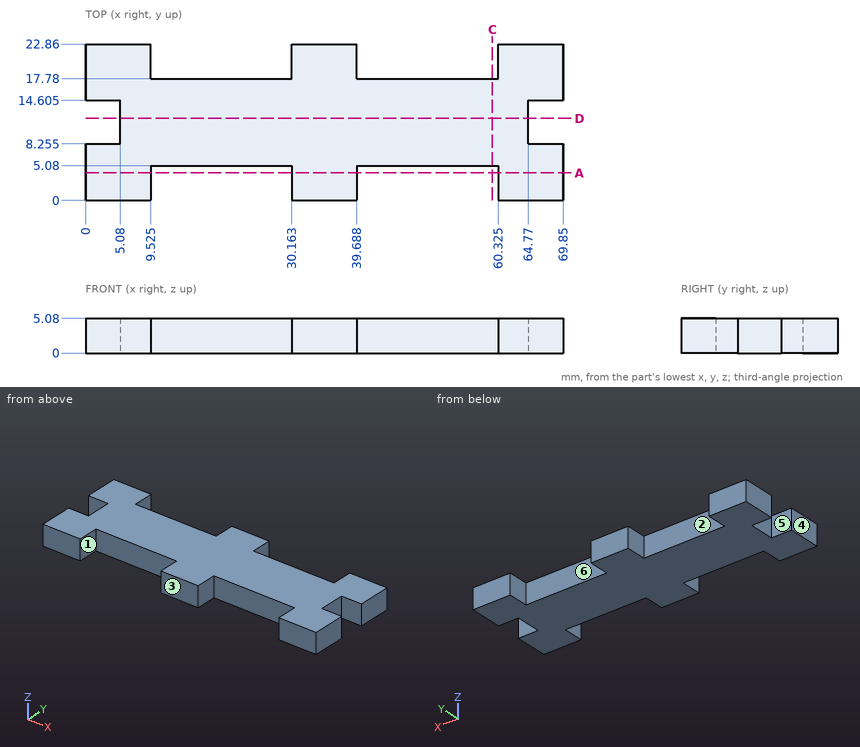
The drawing under review shows one solid part. Ordinate dimensions are in mm from its lowest x, y, z. A direction names the side the tool comes from. Coordinates: 2 decimals unless noted, no trailing zeros. Write each loop counter-clockwise with the first axis right and the second up, starting at its lowest first coordinate (ties: lowest second). Pieces come first, ordered by that corner, then holes. Notation, with made-up numbers: (10, -33.75) -> (15, -33.75) arc R11 ccw to (15, -12.75) -> close; hole circle Ø4 at (45, 30.25). An arc over 180 degrees is marked (long way). One line per item, written item: value. Start each with the question number.
Q1. For the marked faces 1, 2 and 3, list the 3-axis set-ups (+Z, -Z, +X, -X, +Y, -Y) from which the entire face can be reached by the end or side of a thin tool; tool diameter is ignored.
Q2. Add section C-C, the plane x = 59.5. Give the boundary of the cut face in (y, z).
Q3. The part is to be moulded in two halves that separate along X. For the marked faces 4, 5 and 6, say which applies: +X half, -X half, draft (parallel to the pull), parting line (faces both ways), or undercut.
Q4. Add section A-A, the plane y = 4. Count the separate pieces of the cut face and the enclosed holes in it, then the cut area to 3 significant figures.
Q5. Clearance check with flat-ended pins moving along their axes: P1, Ø1.5, axis at x = 1.5, z = 1.5, coming from the -Y side; P2, Ø1, axis at x = 13, z = 2.5, coming from the +Y side; P3, Ø2.5, axis at y = 12.5, z = 3, coming from the -X side; P4, Ø2, axis at x = 29, z = 3.5, coming from the -Y side. State where each tip first meets the part, or that it passes through.
Q6. Add section D-D, the plane y = 12. Give the boundary of the cut face in (x, z).
Q7. To check wall thickness, follow probe 1 along Y at (x, z) = (3.5, 0.75) (1 decimal); probe 2 along Y at (x, z) = (22, 0.6); probe 3 along X at (y, z) = (8.5, 1.35). State the ranges of each line that lie inside material, in increasing order.
Response:
1. face 1: +Z, -Z, -Y
1. face 2: +Z, -Z, +Y
1. face 3: +Z, -Z, +X, -X, -Y
2. outline: (5.08, 0) -> (17.78, 0) -> (17.78, 5.08) -> (5.08, 5.08) -> close
3. face 4: -X half
3. face 5: draft
3. face 6: undercut
4. separate pieces: 3
4. enclosed holes: 0
4. area: 145 mm²
5. P1: y = 0
5. P2: y = 17.78
5. P3: x = 5.08
5. P4: y = 5.08
6. outline: (5.08, 0) -> (64.77, 0) -> (64.77, 5.08) -> (5.08, 5.08) -> close
7. probe 1: 0 to 8.3, 14.6 to 22.9
7. probe 2: 5.08 to 17.78
7. probe 3: 5.08 to 64.77
